```python
from build123d import *

# Parameters (mm, degrees)
F0_R     = 7.85
F1_DEPTH = 3
F2_R     = 4.75
F3_DEPTH = 3


with BuildPart() as f1:
    # F0 (on Front) → F1 (new body)
    with BuildSketch(Plane.XZ):
        Circle(F0_R)
    extrude(amount=F1_DEPTH)

    # F2 (on face) → F3 (join)
    with BuildSketch(Plane.XZ.offset(3)):
        Circle(F2_R)
    extrude(amount=F3_DEPTH)

    # F4 (on Right) → F5 (revolve, cut)
    with BuildSketch(Plane.YZ):
        Polygon((-3.140014, 5.011569), (-1.437357, 7.960658), (0.2653, 5.011569), (1.444096, 8.551884), (-3.541981, 9.199427), align=None)
    revolve(axis=Axis((0, -4.799199, 0), (0, -1, 0)), mode=Mode.SUBTRACT)


solid = f1.part
```
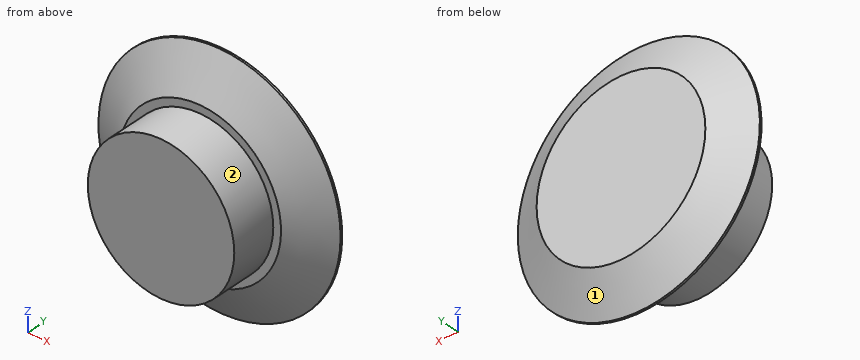
The model under review builds one solid part; all positions refer to its coordinate system, in mm. Face numbers are marked on the shaded views. A direction names the side the tool comes from. Round coordinates to 2 decimals unless told otherwise and drop trailing zeros. Write each loop counter-clockwise with the first axis right and the second up, starting at its lowest first coordinate (ties: lowest second). Pieces come first, ordered by that corner, then holes. Notation, with made-up numbers: (15, 83.5) - (52, 83.5) arc R30 cw to (52, 119.5) - close; hole circle Ø3 at (-13.75, -33.5). An arc over 180 degrees is marked (long way). One line per question, with ' | ' between items.
Item 1: To check wall thickness, follow probe 1 along Y at (x, z) = (-2.75, -4); probe 2 along X at (y, z) = (-4.2, 0.25); probe 3 along Z at (x, y) = (-4, -1.25). State the ranges of each line that lie inside material, in increasing order.
Resolved:
probe 1: y = -3 to 0 | probe 2: x = -4.74 to 4.74 | probe 3: z = -6.5 to 6.5
Item 2: Add section C-C, the plane y = -4.9. Give the boundary of the cut face in (x, z), then the cut area to 3 significant figures.
Resolved:
outline: circle Ø9.5 at (0, 0) | area: 70.9 mm2
Item 3: Add section A-A, the plane z = 0. Give the boundary of the cut face in (x, y), then the cut area to 3 significant figures.
Resolved:
outline: (-7.85, -1.5) - (-5.25, -3) - (-4.75, -3) - (-4.75, -6) - (4.75, -6) - (4.75, -3) - (5.25, -3) - (7.85, -1.5) - (7.85, -1.37) - (5.47, 0) - (-5.47, 0) - (-7.85, -1.37) - close | area: 68.4 mm2
Item 4: Add section D-D, the plane y = -2.2. Give the boundary of the cut face in (x, z), then the cut area to 4 significant figures.
Resolved:
outline: circle Ø13.28 at (0, 0) | area: 138.5 mm2
Item 5: For P1, Ø1, axis at y = -5, z = 2.5, coming from the -X side; P2, Ø2, axis at x = -5.5, y = -2, coming from the +Z side; P3, Ø2, axis at x = -4.5, y = -2, coming from the +Z side, all flat-tipped, find the tip position at first contact; note any pin that passes through.
Resolved:
P1: stops at x = -4.31 | P2: stops at z = 6.34 | P3: stops at z = 6.96
Item 6: Add section B-B, the plane x = 0. Give the boundary of the cut face in (y, z).
Resolved:
outline: (-6, -4.75) - (-3, -4.75) - (-3, -5.25) - (-1.5, -7.85) - (-1.37, -7.85) - (0, -5.47) - (0, 5.47) - (-1.37, 7.85) - (-1.5, 7.85) - (-3, 5.25) - (-3, 4.75) - (-6, 4.75) - close
Item 7: For the marked faces 1 and 2, list the 3-axis set-ups (+Z, -Z, +X, -X, +Y, -Y) from which the entire face can be reached by the end or side of a thin tool; tool diameter is ignored.
Resolved:
face 1: +Y | face 2: -Y
